```python
from build123d import *

# Parameters (mm, degrees)
F0_W     = 175
F0_H     = 76
F0_R     = 3
F1_DEPTH = 25


with BuildPart() as f1:
    # F0 (on Right) → F1 (new body)
    with BuildSketch(Plane.YZ):
        with Locations((-4.577316, 3.653536)):
            Rectangle(F0_W, F0_H)
        with Locations((-68.077316, -22.346464)):
            Circle(F0_R, mode=Mode.SUBTRACT)
        with Locations((66.922684, -22.346464)):
            Circle(F0_R, mode=Mode.SUBTRACT)
        with Locations((-68.077316, 28.653536)):
            Circle(F0_R, mode=Mode.SUBTRACT)
        with Locations((23.922684, 28.653536)):
            Circle(F0_R, mode=Mode.SUBTRACT)
    extrude(amount=F1_DEPTH)


solid = f1.part
```
The model under review builds one solid part; all positions refer to its coordinate system, in mm. Give positions to 0.01 mm unless a question says otherwise; leave off trailing zeros.
(1) For P1, Ø3.5, axis at y = 66.92, z = -22.35, coming from the +X side, flat-tipped, find the tip position at first contact; note if it passes through.
(2) The part is to be moulded in two halves that separate along Y. For faces 1 (the flat face through (12, -6, -34.346)), 2 (the cylindrical face through (12.325, -68.468, 31.628)), 3 (the flat face through (12, 82.923, 3)), say which applies: released by +Y, released by -Y, zero draft, split by the parting line, or undercut.
(3) To check wall thickness, follow L1, parallel to Y at x = 23.25, z = -21; L2, parallel to Y at x = 8.25, z = -20; L3, parallel to Z at x = 18, y = 69. State the ranges of each line that lie inside material, in increasing order.
Returned:
1. P1: passes through
2. face 1: zero draft
2. face 2: undercut
2. face 3: released by +Y
3. L1: y = -92.08 to -70.76, -65.4 to 64.24, 69.6 to 82.92
3. L2: y = -92.08 to -69.95, -66.21 to 65.05, 68.79 to 82.92
3. L3: z = -34.35 to -24.51, -20.18 to 41.65
